The model under review builds one solid part; all positions refer to its coordinate system, in mm. Face numbers are marked on the shaded views. A direction names the side the tool comes from. Coordinates: 2 decimals unless noted, no trailing zeros. Order: outer loops, then holes, each group sorted by start corner. A loop starts at its lowest first (then second) coordinate and runs counter-clockwise, first axis right, second up.
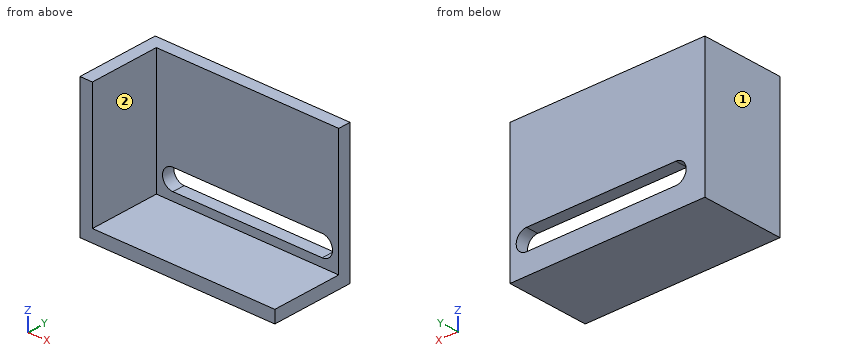
from build123d import *

# Parameters (mm, degrees)
SKETCH2_W           = 44
SKETCH2_H           = 30
BOSS_EXTRUDE1_DEPTH = 3
SKETCH3_W           = 44
SKETCH3_H           = 20
BOSS_EXTRUDE2_DEPTH = 3
SKETCH4_W           = 33
SKETCH4_H           = 20
BOSS_EXTRUDE3_DEPTH = 3
CUT_EXTRUDE1_DEPTH  = 3


with BuildPart() as part:
    # Sketch2 → Boss-Extrude1 (new body)
    with BuildSketch(Plane(origin=(0, 0, 0), x_dir=(1, 0, 0), z_dir=(0, 1, 0))):
        Rectangle(SKETCH2_W, SKETCH2_H)
    extrude(amount=BOSS_EXTRUDE1_DEPTH)

    # Sketch3 → Boss-Extrude2 (add)
    with BuildSketch(Plane(origin=(0, 0, -15), x_dir=(-1, 0, 0), z_dir=(0, 0, -1))):
        with Locations((0, -7)):
            Rectangle(SKETCH3_W, SKETCH3_H)
    extrude(amount=BOSS_EXTRUDE2_DEPTH)

    # Sketch4 → Boss-Extrude3 (add)
    with BuildSketch(Plane.ZY.offset(22)):
        with Locations((-1.5, -7)):
            Rectangle(SKETCH4_W, SKETCH4_H)
    extrude(amount=BOSS_EXTRUDE3_DEPTH)

    # Sketch5 → Cut-Extrude1 (cut)
    with BuildSketch(Plane.XZ):
        with BuildLine():
            Line((-18, -8), (18, -8))
            ThreePointArc((18, -8), (20.5, -10.5), (18, -13))
            Line((18, -13), (-18, -13))
            ThreePointArc((-18, -13), (-20.5, -10.5), (-18, -8))
        make_face()
    extrude(amount=-CUT_EXTRUDE1_DEPTH, mode=Mode.SUBTRACT)


solid = part.part
(1) Tool access review of the marked faces 1 and 2: name each direction out of +Z, -Z, +X, -X, +Y, -Y from which nothing blocks a thin tool from reaching the whole face with its end or side.
(2) Insertion check: pin 1 Ø8.5 at (y, z) = (-11.5, -5) entering from +X; pin 2 Ø10 at (x, z) = (10, 5) entering from -Y. Each pin has a flat end and moves straight along its axis. Give the tip position at first contact, or say it passes through.
(3) Consider section B-B (x = 0). Give the boundary of the cut face in (y, z).
(4) Consider section C-C (z = 6). Give the boundary of the cut face in (x, y).
(5) Wall thickness on line 1 (Z direction, x = 6, y = 0.5); line 2 (Z direction, x = 6, y = -11.5); line 3 (X direction, y = -3.75, z = -12): over which ranges is each line inside the solid? List them lowest first.
(6) Consider section A-A (z = -10.5). Give the boundary of the cut face in (x, y).
(7) Consider section D-D (y = -8.25). Give the boundary of the cut face in (x, z), then the cut area to 3 significant figures.
Findings:
1. face 1: +Z, -Z, -X, +Y, -Y
1. face 2: +Z, +X, -Y
2. pin 1: stops at x = -22
2. pin 2: stops at y = 0
3. outline: (-17, -18) - (3, -18) - (3, -13) - (0, -13) - (0, -15) - (-17, -15) - close; (0, -8) - (3, -8) - (3, 15) - (0, 15) - close
4. outline: (-25, -17) - (-22, -17) - (-22, 0) - (22, 0) - (22, 3) - (-25, 3) - close
5. line 1: z = -18 to -13, -8 to 15
5. line 2: z = -18 to -15
5. line 3: x = -25 to -22
6. outline: (-25, -17) - (-22, -17) - (-22, 0) - (-20.5, 0) - (-20.5, 3) - (-25, 3) - close; (20.5, 0) - (22, 0) - (22, 3) - (20.5, 3) - close
7. outline: (-25, -18) - (22, -18) - (22, -15) - (-22, -15) - (-22, 15) - (-25, 15) - close
7. area: 231 mm2
